Design review of the part built by this model. Coordinates are the model's own, in mm. Face numbers are marked on the shaded views. A direction names the side the tool comes from. Give positions to 0.01 mm unless a question says otherwise; leave off trailing zeros. Order: outer loops, then holes, each group sorted by start corner. A loop starts at its lowest first (then second) coordinate and runs counter-clockwise, first axis right, second up.
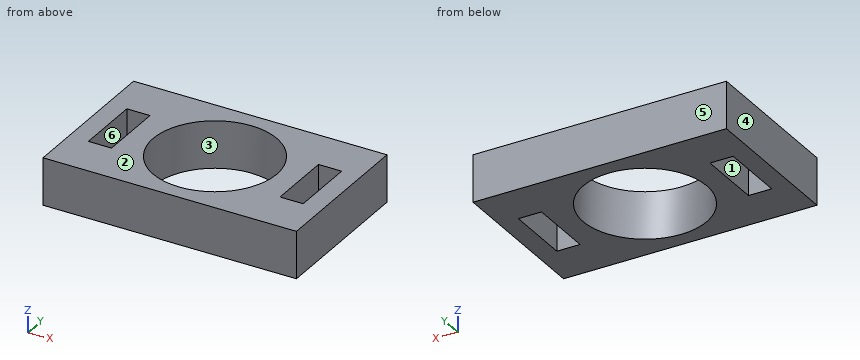
```python
from build123d import *

# Parameters (mm, degrees)
SKETCH1_W           = 32.8
SKETCH1_H           = 20
SKETCH1_R           = 8
SKETCH1_W_2         = 3
SKETCH1_H_2         = 8.5
BOSS_EXTRUDE1_DEPTH = 6.1


with BuildPart() as part:
    # Sketch1 → Boss-Extrude1 (new body)
    with BuildSketch(Plane.XY):
        Rectangle(SKETCH1_W, SKETCH1_H)
        Circle(SKETCH1_R, mode=Mode.SUBTRACT)
        with Locations((12.4, 0)):
            Rectangle(SKETCH1_W_2, SKETCH1_H_2, mode=Mode.SUBTRACT)
        with Locations((-12.4, 0)):
            Rectangle(SKETCH1_W_2, SKETCH1_H_2, mode=Mode.SUBTRACT)
    extrude(amount=BOSS_EXTRUDE1_DEPTH)


solid = part.part
```
1. Take a section at C-C (x = 0). State the section outline as (y, z) points.
Recorded:
outline: (-10, 0) - (-8, 0) - (-8, 6.1) - (-10, 6.1) - close; (8, 0) - (10, 0) - (10, 6.1) - (8, 6.1) - close
2. For pin 1 (9.5 mm diameter, centred on x = 0, y = 0, fed in from -Z), flat-tipped, find the tip position at first contact; note if it passes through.
Recorded:
pin 1: passes through
3. Draft analysis for pull direction X (two halves, no side actions). For the marked faces 1, 2, 3 and 4, state which applies: pulls with the +X half, pulls with the -X half, needs draft (parallel to the pull), parting line crosses it, or undercut.
Recorded:
face 1: undercut
face 2: needs draft
face 3: undercut
face 4: pulls with the -X half
4. Machinability: for the marked faces 5 and 6, which of the approach directions +Z, -Z, +X, -X, +Y, -Y give a long, thin tool a straight path to every point of the face, cutting with its end or side? Answer none if there is none.
Recorded:
face 5: +Z, -Z, +X, -X, +Y
face 6: +Z, -Z
5. For line 1 along X through (y, z) = (0.25, 1.75); line 2 along X through (y, z) = (-1, 4.5); line 3 along Y through (x, z) = (0, 2.25), list the stretches that pass through material, from the lowest coordinate up.
Recorded:
line 1: x = -16.4 to -13.9, -10.9 to -8, 8 to 10.9, 13.9 to 16.4
line 2: x = -16.4 to -13.9, -10.9 to -7.94, 7.94 to 10.9, 13.9 to 16.4
line 3: y = -10 to -8, 8 to 10
6. Take a section at B-B (y = 3.5). State the section outline as (x, z) points, then the cut area to 3 significant figures.
Recorded:
outline: (-16.4, 0) - (-13.9, 0) - (-13.9, 6.1) - (-16.4, 6.1) - close; (-10.9, 0) - (-7.19, 0) - (-7.19, 6.1) - (-10.9, 6.1) - close; (7.19, 0) - (10.9, 0) - (10.9, 6.1) - (7.19, 6.1) - close; (13.9, 0) - (16.4, 0) - (16.4, 6.1) - (13.9, 6.1) - close
area: 75.7 mm2
7. Take a section at D-D (y = -7). State the section outline as (x, z) points.
Recorded:
outline: (-16.4, 0) - (-3.87, 0) - (-3.87, 6.1) - (-16.4, 6.1) - close; (3.87, 0) - (16.4, 0) - (16.4, 6.1) - (3.87, 6.1) - close
8. Take a section at A-A (z = 4). State the section outline as (x, y) points, then the cut area to 3 significant figures.
Recorded:
outline: (-16.4, -10) - (16.4, -10) - (16.4, 10) - (-16.4, 10) - close; hole (-13.9, -4.25) - (-10.9, -4.25) - (-10.9, 4.25) - (-13.9, 4.25) - close; hole circle Ø16 at (0, 0); hole (10.9, -4.25) - (13.9, -4.25) - (13.9, 4.25) - (10.9, 4.25) - close
area: 404 mm2
